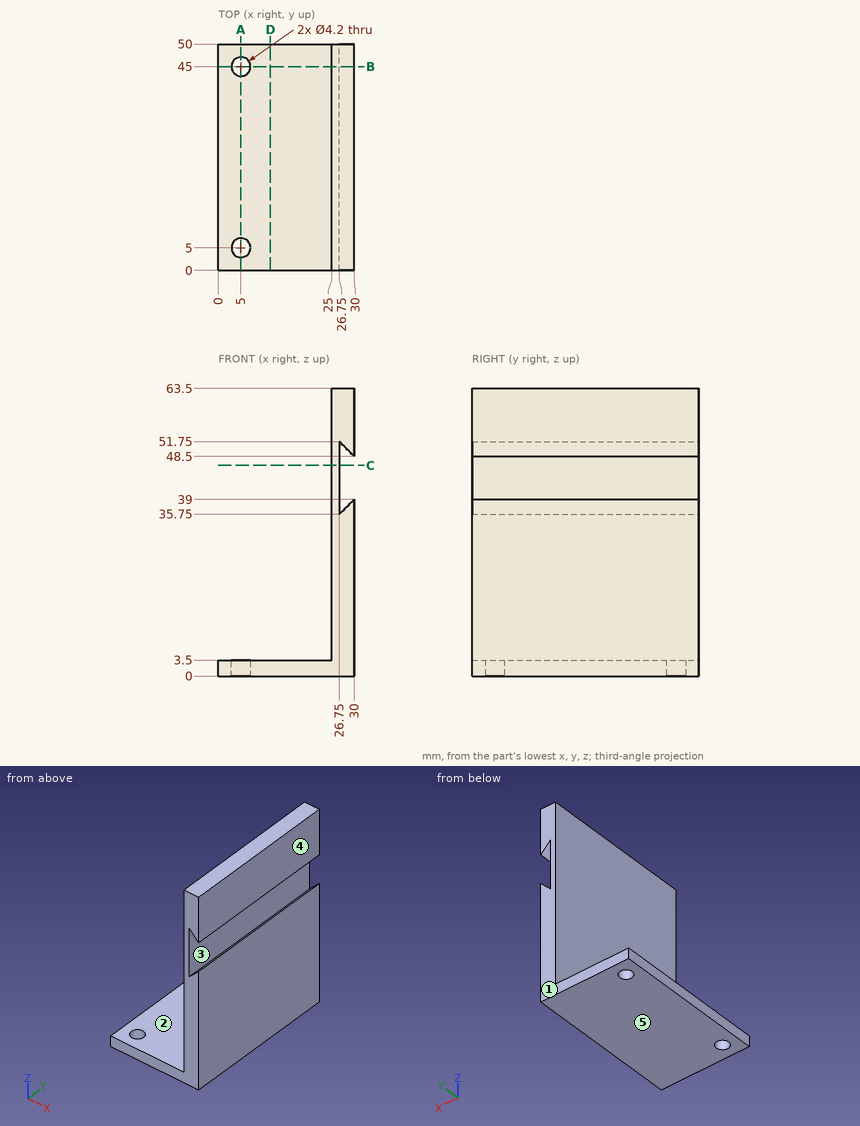
The drawing under review shows one solid part. Ordinate dimensions are in mm from its lowest x, y, z. A direction names the side the tool comes from. Coordinates: 2 decimals unless noted, no trailing zeros. Loops run counter-clockwise (first coordinate to the right, second up) from the corner with the lowest first, then second, coordinate; pieces in that order, holes last. Notation, with made-up numbers: (64, 18) -> (105, 18) arc R28 cw to (105, 48) -> close; hole circle Ø2 at (22.25, -34). An arc over 180 degrees is marked (long way). Answer as a JSON object with one key per item and string values.
Q1. Take a section at C-C on z = 46.5. Give the boundary of the cut face in (x, y), plus the area to 3 significant figures.
Answer block:
{"outline": "(25, 0) -> (26.75, 0) -> (26.75, 50) -> (25, 50) -> close", "area": "87.5 mm^2"}
Q2. Take a section at B-B on y = 45. Give the boundary of the cut face in (x, z), plus the area to 3 significant figures.
Answer block:
{"outline": "(0, 0) -> (2.9, 0) -> (2.9, 3.5) -> (0, 3.5) -> close; (7.1, 0) -> (30, 0) -> (30, 39) -> (26.75, 35.75) -> (26.75, 51.75) -> (30, 48.5) -> (30, 63.5) -> (25, 63.5) -> (25, 3.5) -> (7.1, 3.5) -> close", "area": "349 mm^2"}
Q3. Take a section at D-D on x = 11.5. Give the boundary of the cut face in (y, z).
Answer block:
{"outline": "(0, 0) -> (50, 0) -> (50, 3.5) -> (0, 3.5) -> close"}
Q4. Clearance check with flat-ended pins moving along their axes: pin 1 Ø5 at (x, y) = (14, 34) entering from -Z; pin 2 Ø2 at (x, y) = (22, 30.5) entering from +Z; pin 3 Ø8 at (y, z) = (33, 16) entering from -X. State where each tip first meets the part, or that it passes through.
Answer block:
{"pin 1": "stops at z = 0", "pin 2": "stops at z = 3.5", "pin 3": "stops at x = 25"}
Q5. To check wall thickness, follow L1, parallel to Y at x = 5, z = 1.25; L2, parallel to X at y = 26, z = 59; L3, parallel to Z at x = 22.5, y = 25.5. State the ranges of each line that lie inside material, in increasing order.
Answer block:
{"L1": "y = 0 to 2.9, 7.1 to 42.9, 47.1 to 50", "L2": "x = 25 to 30", "L3": "z = 0 to 3.5"}
Q6. Take a section at A-A on x = 5. Give the boundary of the cut face in (y, z).
Answer block:
{"outline": "(0, 0) -> (2.9, 0) -> (2.9, 3.5) -> (0, 3.5) -> close; (7.1, 0) -> (42.9, 0) -> (42.9, 3.5) -> (7.1, 3.5) -> close; (47.1, 0) -> (50, 0) -> (50, 3.5) -> (47.1, 3.5) -> close"}
Q7. Tool access review of the marked faces 1 and 2: name each direction out of +Z, -Z, +X, -X, +Y, -Y from which nothing blocks a thin tool from reaching the whole face with its end or side.
Answer block:
{"face 1": "+Z, -Z, +X, -X, +Y", "face 2": "+Z, -X, +Y, -Y"}
Q8. The part is to be moulded in two halves that separate along X. For the marked faces 3, 4 and 5, say which applies: +X half, -X half, draft (parallel to the pull), parting line (faces both ways), or undercut.
Answer block:
{"face 3": "undercut", "face 4": "+X half", "face 5": "draft"}
